Here's how the part is built. I have some questions about the finished solid (model axes, mm). Face numbers are marked on the shaded views. A direction names the side the tool comes from. Give positions to 0.01 mm unless a question says otherwise; leave off trailing zeros. Order: outer loops, then holes, each group sorted by start corner. A loop starts at its lowest first (then second) coordinate and runs counter-clockwise, first axis right, second up.
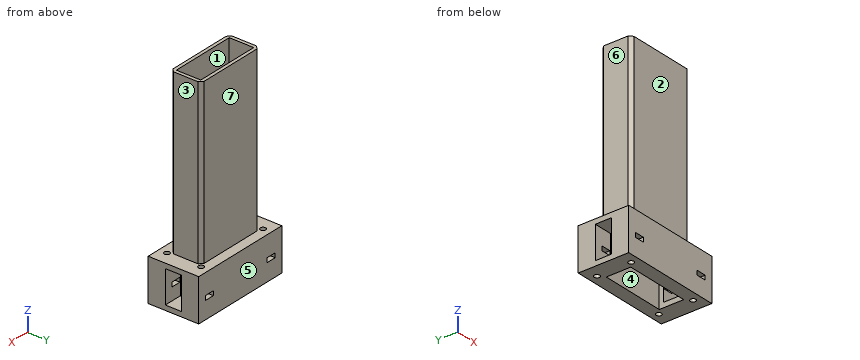
from build123d import *

# Parameters (mm, degrees)
F0_W     = 62.7378050089
F0_H     = 31
F0_W_2   = 40
F0_H_2   = 15
F1_DEPTH = 26
F2_W     = 10
F2_H     = 20
F3_DEPTH = 62.7388050089
F4_D     = 3.3
F5_W     = 44.1129240592
F5_H     = 19
F5_W_2   = 40
F5_H_2   = 15
F6_DEPTH = 100
F7_SIZE  = 2
F8_W     = 6
F8_H     = 2.7
F9_DEPTH = 31.001


with BuildPart() as f1:
    # F0 (on Top) → F1 (new body)
    with BuildSketch(Plane.XY):
        Rectangle(F0_W, F0_H)
        Rectangle(F0_W_2, F0_H_2, mode=Mode.SUBTRACT)
    extrude(amount=F1_DEPTH)

    # F2 (on face) → F3 (cut, through all)
    with BuildSketch(Plane(origin=(-31.3689025044, 0, 0), x_dir=(0, -1, 0), z_dir=(-1, 0, 0))):
        with Locations((0, 13)):
            Rectangle(F2_W, F2_H)
    extrude(amount=-F3_DEPTH, mode=Mode.SUBTRACT)

    # F4 (through all)
    with Locations(Plane(origin=(0, 0, 0), x_dir=(1, 0, 0), z_dir=(0, 0, -1))):
        with Locations((-23.3689025044, -10.5), (-23.3689025044, 10.5), (23.3689025044, 10.5), (23.3689025044, -10.5)):
            Hole(F4_D / 2)

    # F5 (on face) → F6 (join)
    with BuildSketch(Plane.XY.offset(26)):
        Rectangle(F5_W, F5_H)
        Rectangle(F5_W_2, F5_H_2, mode=Mode.SUBTRACT)
    extrude(amount=F6_DEPTH)

    # F7
    f7_edges = [f1.edges().sort_by_distance(p)[0] for p in [
        (22.056462, 9.5, 76),
        (-22.056462, 9.5, 76),
        (22.056462, -9.5, 76),
        (-22.056462, -9.5, 76),
    ]]
    chamfer(f7_edges, length=F7_SIZE)

    # F8 (on face) → F9 (cut, through all)
    with BuildSketch(Plane.XZ.offset(15.5)):
        with Locations((-23.3689025044, 12)):
            Rectangle(F8_W, F8_H)
        with Locations((23.3689025044, 12)):
            Rectangle(F8_W, F8_H)
    extrude(amount=-F9_DEPTH, mode=Mode.SUBTRACT)


solid = f1.part
Q1. If we section it at A-A on z = 19: List the corners of the cut face in (x, y) for me, plus the area to 3 significant figures.
Filled sheet:
outline: (-31.37, -15.5) - (31.37, -15.5) - (31.37, -5) - (20, -5) - (20, -7.5) - (-20, -7.5) - (-20, -5) - (-31.37, -5) - close; (-31.37, 5) - (-20, 5) - (-20, 7.5) - (20, 7.5) - (20, 5) - (31.37, 5) - (31.37, 15.5) - (-31.37, 15.5) - close; hole circle Ø3.3 at (-23.37, -10.5); hole circle Ø3.3 at (-23.37, 10.5); hole circle Ø3.3 at (23.37, -10.5); hole circle Ø3.3 at (23.37, 10.5)
area: 1,080 mm2
Q2. If we section it at B-B on x = 1: List the corners of the cut face in (y, z) for me, plus the area to 3 significant figures.
Filled sheet:
outline: (-15.5, 0) - (-7.5, 0) - (-7.5, 126) - (-9.5, 126) - (-9.5, 26) - (-15.5, 26) - close; (7.5, 0) - (15.5, 0) - (15.5, 26) - (9.5, 26) - (9.5, 126) - (7.5, 126) - close
area: 816 mm2
Q3. I'm going to push flat-ended pins straight in: P1, Ø5, axis at x = 24, y = -10.5, coming from the +Z side; P2, Ø12, axis at y = -8.5, z = 50, coming from the -X side; P3, Ø1, axis at x = -5.5, z = 41, coming from the -Y side; P4, Ø5, axis at x = -24.5, y = 1, coming from the +Z side. Where does each tip first touch, or does it pass through?
Filled sheet:
P1: stops at z = 26
P2: stops at x = -22.06
P3: stops at y = -9.5
P4: stops at z = 126
Q4. Thinking about a two-plate mould opening in X: for the marked faces 1, 2 and 3, which applies, released by +X, released by -X, zero draft, split by the parting line, or undercut?
Filled sheet:
face 1: undercut
face 2: zero draft
face 3: released by +X
Q5. I need wall thicknesses on L1, parallel to X at y = -10.5, z = 17.75; L2, parallel to Z at x = -20.5, y = 0; L3, parallel to Y at x = 5, z = 90. Which ranges of each line are inside material? Lowest first, please.
Filled sheet:
L1: x = -31.37 to -25.02, -21.72 to 21.72, 25.02 to 31.37
L2: z = 0 to 3, 23 to 126
L3: y = -9.5 to -7.5, 7.5 to 9.5
Q6. If we section it at D-D on z = 72: List the corners of the cut face in (x, y) for me, plus the area to 3 significant figures.
Filled sheet:
outline: (-22.06, -7.5) - (-20.06, -9.5) - (20.06, -9.5) - (22.06, -7.5) - (22.06, 7.5) - (20.06, 9.5) - (-20.06, 9.5) - (-22.06, 7.5) - close; hole (-20, -7.5) - (20, -7.5) - (20, 7.5) - (-20, 7.5) - close
area: 230 mm2
Q7. If we section it at C-C on y = 3: List the corners of the cut face in (x, z) for me, plus the area to 3 significant figures.
Filled sheet:
outline: (-31.37, 0) - (-20, 0) - (-20, 3) - (-31.37, 3) - close; (-31.37, 23) - (-20, 23) - (-20, 126) - (-22.06, 126) - (-22.06, 26) - (-31.37, 26) - close; (20, 0) - (31.37, 0) - (31.37, 3) - (20, 3) - close; (20, 23) - (31.37, 23) - (31.37, 26) - (22.06, 26) - (22.06, 126) - (20, 126) - close
area: 548 mm2
Q8. For the marked faces 4, 5, 6 and 7, which set-ups out of +Z, -Z, +X, -X, +Y, -Y let a thin tool reach every point of the face, with its end or its side?
Filled sheet:
face 4: +Z, -Z
face 5: +Z, -Z, +X, -X, +Y
face 6: +Z, -X, +Y, -Y
face 7: +Z, +X, -X, +Y
